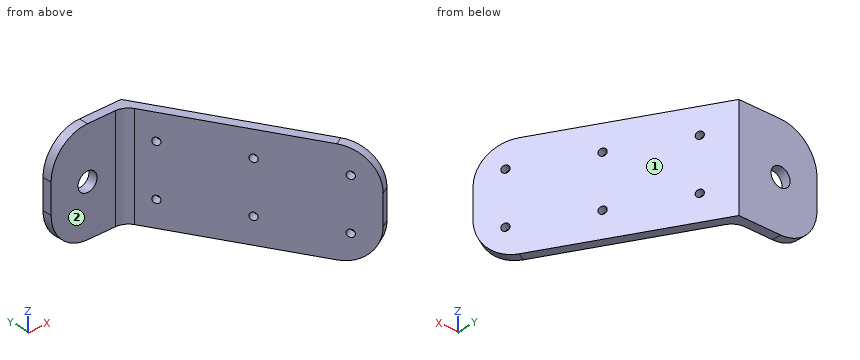
Autodesk Inventor part; units mm, degrees
ref_plane "YZ Plane" through (0, 0, 0) normal (1, 0, 0) x (0, 1, 0)
ref_plane "XZ Plane" through (0, 0, 0) normal (0, 1, 0) x (-1, 0, 0)
ref_plane "XY Plane" through (0, 0, 0) normal (0, 0, 1) x (1, 0, 0)
sketch "Sketch1" plane through (0, 0, 0) normal (0, 0, 1) x (1, 0, 0)
  line L0 (13.3846, -4.4923) -> (-12.0154, -4.4923)
  line L1 (-12.0154, -1.3173) -> (-12.0154, -4.4923)
  line L2 (13.3846, -4.4923) -> (84.5046, -4.4923) construction
  line L3 (13.3846, -4.4923) -> (84.5046, -4.4923) construction
  line L4 (13.3846, -4.4923) -> (84.5046, -4.4923) construction
  line L5 (13.3846, -4.4923) -> (48.9446, -66.084)
  line L6 (13.3846, -4.4923) -> (84.5046, -4.4923) construction
  line L7 (48.9446, -66.084) -> (51.6943, -64.4965)
  line L8 (-12.0154, -1.3173) -> (15.2177, -1.3173)
  line L9 (51.6943, -64.4965) -> (15.2177, -1.3173)
  dimension "d13" = 3.175
  dimension "d30" = 71.12
  dimension "d31" = 60
  dimension "d32" = 3.175
extrude "Extrusion1" add sketch "Sketch1" along normal blind 35.56
sketch "Sketch2" plane through (-12.0154, -1.3173, 0) normal (0, 1, 0) x (1, 0, 0)
  line L0 (0, 0) -> (27.2331, 0)
  line L1 (0, 0) -> (0, -35.56)
  point P0 (12.0154, 0)
  point P1 (12.7, -17.78)
  dimension "d45" = 17.78
  dimension "d46" = 12.7
hole "Hole1" at (0.6846, -1.3173, 17.78) direction (0, -1, 0) diameter 6.604 depth 3.175 tip angle 118
sketch "Sketch3" plane through (15.2177, -1.3173, 35.56) normal (0.866, 0.5, 0) x (0, 0, -1)
  line L0 (35.56, -72.9531) -> (0, -72.9531)
  line L1 (35.56, 0) -> (35.56, -72.9531)
  point P0 (35.56, 8.7496)
  point P1 (26.67, -64.0631)
  dimension "d47" = 8.89
  dimension "d48" = 8.89
hole "Hole2" at (47.2493, -56.7975, 8.89) direction (-0.866, -0.5, 0) diameter 2.54 depth 3.175 tip angle 118
sketch "Sketch4" plane through (15.2177, -1.3173, 35.56) normal (0.866, 0.5, 0) x (0, 0, -1)
  line L0 (0, -72.9531) -> (0, 0)
  line L1 (35.56, -72.9531) -> (0, -72.9531)
  point P0 (35.56, 8.7496)
  point P1 (8.89, -64.0631)
  dimension "d56" = 8.89
  dimension "d57" = 8.89
hole "Hole3" at (47.2493, -56.7975, 26.67) direction (-0.866, -0.5, 0) diameter 2.54 depth 3.175 tip angle 118
sketch "Sketch5" plane through (15.2177, -1.3173, 35.56) normal (0.866, 0.5, 0) x (0, 0, -1)
  line L0 (0, -72.9531) -> (0, 0)
  line L1 (35.56, -72.9531) -> (0, -72.9531)
  point P0 (35.56, 8.7496)
  point P1 (8.89, -37.3931)
  dimension "d65" = 8.89
  dimension "d66" = 35.56
hole "Hole4" at (33.9143, -33.7006, 26.67) direction (-0.866, -0.5, 0) diameter 2.54 depth 3.175 tip angle 118
sketch "Sketch6" plane through (15.2177, -1.3173, 35.56) normal (0.866, 0.5, 0) x (0, 0, -1)
  line L0 (35.56, 0) -> (35.56, -72.9531)
  line L1 (35.56, -72.9531) -> (0, -72.9531)
  point P0 (35.56, 8.7496)
  point P1 (26.67, -37.3931)
  dimension "d74" = 8.89
  dimension "d75" = 35.56
hole "Hole5" at (33.9143, -33.7006, 8.89) direction (-0.866, -0.5, 0) diameter 2.54 depth 3.175 tip angle 118
sketch "Sketch7" plane through (15.2177, -1.3173, 35.56) normal (0.866, 0.5, 0) x (0, 0, -1)
  line L0 (35.56, 0) -> (35.56, -72.9531)
  line L1 (35.56, 0) -> (0, 0)
  circle A0 centre (26.67, -37.3931) radius 1.27
  point P0 (35.56, 8.7496)
  point P1 (26.67, -10.7231)
  dimension "d83" = 8.89
  dimension "d101" = 26.67
hole "Hole6" at (20.5793, -10.6037, 8.89) direction (-0.866, -0.5, 0) diameter 2.54 depth 3.175 tip angle 118
sketch "Sketch8" plane through (15.2177, -1.3173, 35.56) normal (0.866, 0.5, 0) x (0, 0, -1)
  line L0 (35.56, 0) -> (0, 0)
  line L1 (0, -72.9531) -> (0, 0)
  circle A0 centre (8.89, -37.3931) radius 1.27
  point P0 (35.56, 8.7496)
  point P1 (8.89, -10.7231)
  dimension "d93" = 8.89
  dimension "d102" = 26.67
hole "Hole7" at (20.5793, -10.6037, 26.67) direction (-0.866, -0.5, 0) diameter 2.54 depth 3.175 tip angle 118
fillet "Fillet1" radius 12.7 1 edges at (50.3194, -65.2902, 0)
fillet "Fillet2" radius 12.7 1 edges at (50.3194, -65.2902, 35.56)
fillet "Fillet3" radius 12.7 1 edges at (-12.0154, -2.9048, 35.56)
fillet "Fillet4" radius 12.7 1 edges at (-12.0154, -2.9048, 0)
fillet "Fillet5" radius 5.08 1 edges at (13.3846, -4.4923, 17.78)
properties part number "matrix_holder"
For this review, take the finished solid that the model builds, in its own axes (mm). Face numbers are marked on the shaded views. A direction names the side the tool comes from. Give positions to 0.01 mm unless a question says otherwise; leave off trailing zeros. Loops run counter-clockwise (first coordinate to the right, second up) from the corner with the lowest first, then second, coordinate; pieces in that order, holes last. Notation, with made-up numbers: M 69.5,89.5 L 82.5,89.5 A4 ccw 82.5,95.5 Z; hole C 61.5,-22 d3. An arc over 180 degrees is marked long. Answer as a JSON object with one key per item and string values. Group by question number.
Q1. Add section D-D on y = -5.5. Give the boundary of the cut face in (x, z), and give its area (3 significant figures).
Q2. For probe 1 along Z at (x, y) = (18.5, -11.5); probe 2 along Y at (x, z) = (5, 31.5); probe 3 along X at (y, z) = (-3, 17), list the stretches that pass through material, from the lowest coordinate up. Write a range as [from, to].
Q3. Add section A-A on z = 17.78. Give the boundary of the cut face in (x, y), and give its area (3 significant figures).
Q4. Add section B-B on x = 6. Give the boundary of the cut face in (y, z).
Q5. Tool access review of the marked faces 1 and 2: name each direction out of +Z, -Z, +X, -X, +Y, -Y from which nothing blocks a thin tool from reaching the whole face with its end or side.
Q6. Insertion check: P1, Ø1.5, axis at y = -9, z = 20.5, coming from the -X side; P2, Ø1, axis at y = -14, z = 18, coming from the +X side; P3, Ø1, axis at y = -34, z = 13, coming from the -X side; P4, Ø10.5, axis at x = 0.68, z = 17.78, coming from the +Y side. Each pin has a flat end and moves straight along its axis. Give the tip position at first contact, or say it passes through.
Q7. Add section C-C on z = 4.5. Give the boundary of the cut face in (x, y).
Checked values:
{
 "1": {"outline": "M 13.49,0 L 17.63,0 L 17.63,35.56 L 13.49,35.56 Z", "area": "147 mm²"},
 "2": {"probe 1": "[0, 7.65], [10.13, 25.43], [27.91, 35.56]", "probe 2": "[-4.49, -1.32]", "probe 3": "[-12.02, -2.52], [3.89, 16.19]"},
 "3": {"outline": "M -12.02,-4.49 L -2.62,-4.49 L -2.62,-1.32 L -12.02,-1.32 Z; M 3.99,-4.49 L 10.45,-4.49 A5.08 cw 14.85,-7.03 L 48.94,-66.08 L 51.69,-64.5 L 15.22,-1.32 L 3.99,-1.32 Z", "area": "293 mm²"},
 "4": {"outline": "M -4.49,0 L -1.32,0 L -1.32,35.56 L -4.49,35.56 Z"},
 "5": {"face 1": "+Z, -Z, +X, +Y", "face 2": "+Z, -Z, -X, -Y"},
 "6": {"P1": "x = 15.55", "P2": "x = 22.83", "P3": "x = 30.13", "P4": "y = -1.32"},
 "7": {"outline": "M -9.01,-4.49 L 10.45,-4.49 A5.08 cw 14.85,-7.03 L 47.44,-63.48 L 50.19,-61.9 L 15.22,-1.32 L -9.01,-1.32 Z"}
}
